```python
from build123d import *

# Parameters (mm, degrees)
BOSS_EXTRUDE1_DEPTH      = 63.5
BOSS_EXTRUDE1_DEPTH_BACK = 63.5
SKETCH3_W                = 12.7
SKETCH3_H                = 6.35
BOSS_EXTRUDE2_DEPTH      = 63.5
BOSS_EXTRUDE2_DEPTH_BACK = 63.5
SKETCH4_W                = 12.7
SKETCH4_H                = 6.35
CUT_EXTRUDE2_DEPTH       = 161.809264194
CUT_EXTRUDE2_DEPTH_BACK  = 161.809264194
SKETCH5_R                = 50.8
FILLET1_R                = 2.54


with BuildPart() as part:
    # Sketch2 → Revolve1 (revolve)
    with BuildSketch(Plane.YZ, mode=Mode.PRIVATE) as revolve1_sk:
        with BuildLine():
            Line((-76.2, -119.359706143), (-76.2, -5.059706143))
            Line((-76.2, -5.059706143), (-63.435713245, -5.059706143))
            ThreePointArc((-63.435713245, -5.059706143), (-60.260713245, -1.884706143), (-63.435713245, 1.290293857))
            Line((-63.435713245, 1.290293857), (-69.785713245, 1.290293857))
            Line((-69.785713245, 1.290293857), (-69.785713245, 7.640293857))
            Line((-69.785713245, 7.640293857), (-63.5, 7.640293857))
            ThreePointArc((-63.5, 7.640293857), (-60.325, 10.815293857), (-63.5, 13.990293857))
            Line((-63.5, 13.990293857), (-69.85, 13.990293857))
            Line((-69.85, 13.990293857), (-69.85, 20.340293857))
            Line((-69.85, 20.340293857), (-57.15, 20.340293857))
            Line((-57.15, 20.340293857), (-57.15, 33.040293857))
            Line((-57.15, 33.040293857), (-50.8, 33.040293857))
            Line((-50.8, 33.040293857), (-50.8, -11.409706143))
            Line((-50.8, -11.409706143), (-63.5, -11.409706143))
            Line((-63.5, -11.409706143), (-63.5, -81.259706143))
            Line((-63.5, -81.259706143), (-69.785713245, -81.259706143))
            Line((-69.785713245, -81.259706143), (-69.785713245, -119.359706143))
            Line((-69.785713245, -119.359706143), (-76.2, -119.359706143))
        make_face()
    revolve(revolve1_sk.sketch.rotate(Axis((0, 0, 44.403866564), (0, 0, -1)), 270), axis=Axis((0, 0, 44.403866564), (0, 0, -1)))

    # Sketch3 → Boss-Extrude1 (add, two sides: drawn at the far end of the back side and taken through both)
    with BuildSketch(Plane.YZ.offset(-BOSS_EXTRUDE1_DEPTH_BACK)):
        with Locations((0, 29.865293857)):
            Rectangle(SKETCH3_W, SKETCH3_H)
    extrude(amount=BOSS_EXTRUDE1_DEPTH + BOSS_EXTRUDE1_DEPTH_BACK)

    # Sketch4 → Boss-Extrude2 (add, two sides: drawn at the far end of the back side and taken through both)
    with BuildSketch(Plane(origin=(0, 0, 0), x_dir=(-1, 0, 0), z_dir=(0, 1, 0)).offset(-BOSS_EXTRUDE2_DEPTH_BACK)):
        with Locations((0, 29.865293857)):
            Rectangle(SKETCH4_W, SKETCH4_H)
    extrude(amount=BOSS_EXTRUDE2_DEPTH + BOSS_EXTRUDE2_DEPTH_BACK)

    # Sketch5 → Cut-Extrude2 (cut, two sides: drawn at the far end of the back side and taken through both)
    with BuildSketch(Plane(origin=(0, 0, 0), x_dir=(0, 1, 0), z_dir=(0, 0, 1)).offset(-CUT_EXTRUDE2_DEPTH_BACK)):
        with Locations(Location((0, 0, 0), (0, 0, 270))):
            Circle(SKETCH5_R)
    extrude(amount=CUT_EXTRUDE2_DEPTH + CUT_EXTRUDE2_DEPTH_BACK, mode=Mode.SUBTRACT)

    # Fillet1
    fillet1_edges = [part.edges().sort_by_distance(p)[0] for p in [
        (6.35, 63.5, 29.865293857),
        (0, 63.5, 26.690293857),
        (-6.35, 63.5, 29.865293857),
        (0, 63.5, 33.040293857),
        (-63.5, -6.35, 29.865293857),
        (-63.5, 0, 33.040293857),
        (-63.5, 6.35, 29.865293857),
        (-63.5, 0, 26.690293857),
        (63.5, -6.35, 29.865293857),
        (63.5, 0, 26.690293857),
        (63.5, 6.35, 29.865293857),
        (63.5, 0, 33.040293857),
        (6.35, -63.5, 29.865293857),
        (0, -63.5, 33.040293857),
        (-6.35, -63.5, 29.865293857),
        (0, -63.5, 26.690293857),
    ]]
    fillet(fillet1_edges, radius=FILLET1_R)


solid = part.part
```
Geometry check sheet. Reference: the model listing, model coordinates, mm. A direction names the side the tool comes from. Coordinates: 2 decimals unless noted, no trailing zeros. Write each loop counter-clockwise with the first axis right and the second up, starting at its lowest first coordinate (ties: lowest second). Pieces come first, ordered by that corner, then holes. Notation, with made-up numbers: M 7.5,9 L 53.5,9 A11 cw 53.5,28 Z; hole C -27,-37.5 d9. An arc over 180 degrees is marked long. Use one line per item in the form item = value. Start each with the question number.
1) Set-up check for faces 1 (the flat face through (-6.35, 59, 30)), 2 (the flat face through (-6.35, -59, 30)), 3 (the cylindrical face through (-15.1, 68.2, 17.2)): record each of +Z, -Z, +X, -X, +Y, -Y from which the full face is reachable in a straight line by a thin tool's end or side.
2) Release check for a two-part mould opening along Y. For faces 4 (the cylindrical face through (-40.313, -30.911, 10.504)), 5 (the cylindrical face through (-13.77, 61.99, -46.82)), 6 (the flat face through (-15, 62, 1.29)), 7 (the flat face through (-59, 6.35, 30)) record: pulls with the +Y half, pulls with the -Y half, needs draft (parallel to the pull), parting line crosses it, or undercut.
3) Thickness scan on probe 1 along Z at (x, y) = (26, 58.5); probe 2 along Y at (x, z) = (0, -110); probe 3 along Z at (x, y) = (-57.5, 2). Record the ranges inside material, lowest first. Write a range as from..to.
4) Section check B-B on z = -110. Enter the section's corners in (x, y), and give its area (3 significant figures).
5) Go/stop test with flat-tipped pins: pin 1 Ø10 at (y, z) = (8, -80) entering from +X; pin 2 Ø4.5 at (y, z) = (59.5, 30) entering from -X; pin 3 Ø10 at (x, y) = (45, 21.5) entering from -Z. Record where each tip stops, or that it passes through.
6) Section check A-A on z = -40.5. Enter the section's corners in (x, y).
Responses:
q1.face_1 = +Z, -X, +Y
q1.face_2 = +Z, -X, -Y
q1.face_3 = +Z
q2.face_4 = undercut
q2.face_5 = undercut
q2.face_6 = needs draft
q2.face_7 = pulls with the +Y half
q3.probe_1 = -81.26..-5.06, 1.29..7.64, 13.99..20.34
q3.probe_2 = -76.2..-69.79, 69.79..76.2
q3.probe_3 = -11.41..20.34, 26.69..33.04
q4.outline = C 0,0 d152.4; hole C 0,0 d139.57
q4.area = 2,940 mm2
q5.pin_1 = 76.14
q5.pin_2 = -6.35
q5.pin_3 = -11.41
q6.outline = C 0,0 d152.4; hole C 0,0 d127
